```python
from build123d import *

# Parameters (mm, degrees)
F0_W     = 5.08
F0_H     = 50.8
F0_W_2   = 2.54
F0_H_2   = 38.1
F1_DEPTH = 10.16
F2_DEPTH = 5.08
F3_R     = 1.27
F4_DEPTH = 2.54


with BuildPart() as f1:
    # F0 (on Top) → F1 (new body)
    with BuildSketch(Plane.XY):
        with Locations((-11.560145, 0.263519)):
            Rectangle(F0_W, F0_H)
        with Locations((-11.560145, 1.533519)):
            Rectangle(F0_W_2, F0_H_2, mode=Mode.SUBTRACT)
        with Locations((-11.560145, 1.533519)):
            Rectangle(F0_W_2, F0_H_2)
    extrude(amount=F1_DEPTH)

    # F0 (on Top) → F2 (cut)
    with BuildSketch(Plane.XY):
        with Locations((-11.560145, 1.533519)):
            Rectangle(F0_W_2, F0_H_2)
    extrude(amount=F2_DEPTH, mode=Mode.SUBTRACT)

    # F3 (on face) → F4 (join)
    with BuildSketch(Plane(origin=(-10.290145, 0, 0), x_dir=(0, -1, 0), z_dir=(-1, 0, 0))):
        with Locations((-18.043519, 2.54)):
            Circle(F3_R)
    extrude(amount=F4_DEPTH)


solid = f1.part
```
The listing builds one solid part. Answer for the finished solid, in the listing's coordinates (mm). A direction names the side the tool comes from. Round coordinates to 2 decimals unless told otherwise and drop trailing zeros. Loops run counter-clockwise (first coordinate to the right, second up) from the corner with the lowest first, then second, coordinate; pieces in that order, holes last.
Q1. Section C-C, the plane y = -7 is taken. Determine the outline of the cut face in (x, z).
Q2. Section A-A, the plane x = -11.8 is taken. Determine the outline of the cut face in (y, z), then the cut area to 3 significant figures.
Q3. Which of the six approach directions +Z, -Z, +X, -X, +Y, -Y give full straight-line access (tool end or side, diameter ignored) to faces 4 (the face through (-12, 20.584, 3)), 5 (the face through (-11.54, 18.32, 1.3)), 6 (the face through (-12, 1, 10.16))?
Q4. Find the intervals of material crossed by line 1 (Y direction, x = -11.1, z = 4.25); line 2 (X direction, y = -5.5, z = 2.25); line 3 (Y direction, x = -10.45, z = 3.5), in increasing order.
Q5. Section B-B, the plane z = 2.54 is taken. Determine the outline of the cut face in (x, y).
Q6. Given pin 1 Ø1 at (x, y) = (-12, -9) entering from -Z, flat-ended and moving along its own axis, determine where the tip first touches the part or whether it passes through.
Q7. For a pull along X with two mould halves and no side action, classify faces 1 (the face through (-14.1, 0, 5)), 2 (the face through (-12, -17.516, 3)), 3 (the face through (-12, -25.136, 5)) as released by +X, released by -X, zero draft, split by the parting line, or undercut.
Completed:
1. outline: (-14.1, 0) - (-12.83, 0) - (-12.83, 5.08) - (-10.29, 5.08) - (-10.29, 0) - (-9.02, 0) - (-9.02, 10.16) - (-14.1, 10.16) - close
2. outline: (-25.14, 0) - (-17.52, 0) - (-17.52, 5.08) - (20.58, 5.08) - (20.58, 0) - (25.66, 0) - (25.66, 10.16) - (-25.14, 10.16) - close; circle Ø2.54 at (18.04, 2.54)
2. area: 328 mm2
3. face 4: -Z
3. face 5: none
3. face 6: +Z, +X, -X, +Y, -Y
4. line 1: y = -25.14 to -17.52, 20.58 to 25.66
4. line 2: x = -14.1 to -12.83, -10.29 to -9.02
4. line 3: y = -25.14 to -17.52, 17.21 to 18.87, 20.58 to 25.66
5. outline: (-14.1, -25.14) - (-9.02, -25.14) - (-9.02, 25.66) - (-14.1, 25.66) - close; hole (-12.83, -17.52) - (-10.29, -17.52) - (-10.29, 16.77) - (-12.83, 16.77) - close; hole (-12.83, 19.31) - (-10.29, 19.31) - (-10.29, 20.58) - (-12.83, 20.58) - close
6. pin 1: stops at z = 5.08
7. face 1: released by -X
7. face 2: undercut
7. face 3: zero draft
